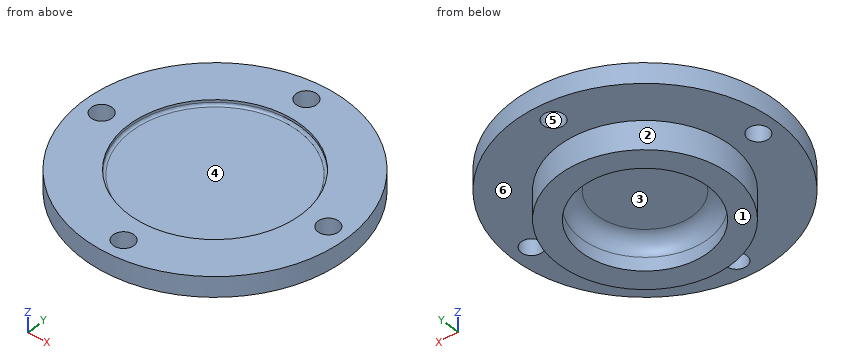
from build123d import *

# Parameters (mm, degrees)
SKETCH_1_R          = 52
SKETCH_1_R_2        = 4.1
EXTRUDE_1_DEPTH     = 8
SKETCH_2_R          = 34
CUT_EXTRUDE_1_DEPTH = 2
FILLET_1_R          = 1
SKETCH_3_R          = 34
SKETCH_3_R_2        = 25
EXTRUDE_2_DEPTH     = 11.3
FILLET_2_R          = 6


with BuildPart() as part:
    # Эскиз1 → Бобышка-Вытянуть1 (new body)
    with BuildSketch(Plane.XY):
        Circle(SKETCH_1_R)
        with Locations((0, 44)):
            Circle(SKETCH_1_R_2, mode=Mode.SUBTRACT)
        with Locations((44, 0)):
            Circle(SKETCH_1_R_2, mode=Mode.SUBTRACT)
        with Locations((0, -44)):
            Circle(SKETCH_1_R_2, mode=Mode.SUBTRACT)
        with Locations((-44, 0)):
            Circle(SKETCH_1_R_2, mode=Mode.SUBTRACT)
    extrude(amount=EXTRUDE_1_DEPTH)

    # Эскиз2 → Вырез-Вытянуть1 (cut)
    with BuildSketch(Plane.XY.offset(8)):
        Circle(SKETCH_2_R)
    extrude(amount=-CUT_EXTRUDE_1_DEPTH, mode=Mode.SUBTRACT)

    # Скругление1
    fillet_1_edges = [part.edges().sort_by_distance(p)[0] for p in [
        (-34, 0, 6),
    ]]
    fillet(fillet_1_edges, radius=FILLET_1_R)

    # Эскиз3 → Бобышка-Вытянуть2 (add)
    with BuildSketch(Plane(origin=(0, 0, 0), x_dir=(-1, 0, 0), z_dir=(0, 0, -1))):
        with Locations(Location((0, 0, 0), (0, 0, 180))):
            Circle(SKETCH_3_R)
        Circle(SKETCH_3_R_2, mode=Mode.SUBTRACT)
    extrude(amount=EXTRUDE_2_DEPTH)

    # Скругление2
    fillet_2_edges = [part.edges().sort_by_distance(p)[0] for p in [
        (25, 0, 0),
    ]]
    fillet(fillet_2_edges, radius=FILLET_2_R)


solid = part.part
Work out the finished part from the listing and answer in its coordinate system (mm). Face numbers are marked on the shaded views. A direction names the side the tool comes from. Give positions to 0.01 mm unless a question says otherwise; leave off trailing zeros. Loops run counter-clockwise (first coordinate to the right, second up) from the corner with the lowest first, then second, coordinate; pieces in that order, holes last. Notation, with made-up numbers: M -37,1.5 L -5,1.5 A11 cw -5,7.5 Z; hole C -20,-38 d7. An arc over 180 degrees is marked long. Use CSV: the item, a comma, the result in double quotes.
1) Find section A-A on y = 0. Write down the section's boundary in (x, z).
Answer:
outline,"M -52,0 L -48.1,0 L -48.1,8 L -52,8 Z; M -39.9,0 L -34,0 L -34,-11.3 L -25,-11.3 L -25,-6 A6 cw -19,0 L 19,0 A6 cw 25,-6 L 25,-11.3 L 34,-11.3 L 34,0 L 39.9,0 L 39.9,8 L 34,8 L 34,7 A1 cw 33,6 L -33,6 A1 cw -34,7 L -34,8 L -39.9,8 Z; M 48.1,0 L 52,0 L 52,8 L 48.1,8 Z"
2) Find section C-C on y = -44. Write down the section's boundary in (x, z), plus the area to 3 significant figures.
Answer:
outline,"M -27.71,0 L -4.1,0 L -4.1,8 L -27.71,8 Z; M 4.1,0 L 27.71,0 L 27.71,8 L 4.1,8 Z"
area,"378 mm^2"
3) Given P1, Ø2, axis at x = 29, z = -8.5, coming from the -Y side; P2, Ø2, axis at y = -10.5, z = -3.5, coming from the -X side; P3, Ø1, axis at y = 10.5, z = -7.5, coming from the +X side, each flat-ended and moving along its own axis, determine where each tip first touches the part or whether it passes through.
Answer:
P1,"y = -19.29"
P2,"x = -32.65"
P3,"x = 32.5"
4) Which of the six approach directions +Z, -Z, +X, -X, +Y, -Y give full straight-line access (tool end or side, diameter ignored) to the marked faces 5 and 6?
Answer:
face 5,"+Z, -Z"
face 6,"-Z"
5) Determine the mould class of the marked faces 1, 2, 3 and 4 for opening direction X: released by +X, released by -X, zero draft, split by the parting line, or undercut.
Answer:
face 1,"zero draft"
face 2,"split by the parting line"
face 3,"undercut"
face 4,"undercut"
6) Consider L1, parallel to Y at x = 0, z = 3; L2, parallel to Z at x = -21, y = 47; L3, parallel to Y at x = 44, z = 3. Determine where each line is inside the solid, lowest interval first.
Answer:
L1,"-52 to -48.1, -39.9 to 39.9, 48.1 to 52"
L2,"0 to 8"
L3,"-27.71 to -4.1, 4.1 to 27.71"
